from build123d import *

# Parameters (mm, degrees)
CUT_EXTRUDE_START        = -5
SKETCH_2_R               = 1.75
CUT_EXTRUDE_1_DEPTH      = 39.496268449
SKETCH_4_W               = 1.25
SKETCH_4_H               = 8
PATTERN_CIRCULAR_1_COUNT = 2
PATTERN_CIRCULAR_1_ANGLE = 90


with BuildPart() as part:
    # ｽｹｯﾁ1 → 回転1 (revolve)
    with BuildSketch(Plane.XY, mode=Mode.PRIVATE) as revolve_1_sk:
        with BuildLine():
            Line((5, 16), (5, 3))
            Line((5, 3), (-5, 3))
            Line((-5, 3), (-5, 16))
            Line((-5, 16), (-2.886751346, 16))
            Line((-2.886751346, 16), (-1.732050808, 14))
            ThreePointArc((-1.732050808, 14), (0, 13), (1.732050808, 14))
            Line((1.732050808, 14), (2.886751346, 16))
            Line((2.886751346, 16), (5, 16))
        make_face()
    revolve(revolve_1_sk.sketch.rotate(Axis((-76.157807816, 0, 0), (1, 0, 0)), 90), axis=Axis((-76.157807816, 0, 0), (1, 0, 0)))

    # ｽｹｯﾁ2 → ｶｯﾄ - 押し出し1 (cut)
    with BuildSketch(Plane(origin=(0, 13, 0), x_dir=(1, 0, 0), z_dir=(0, 1, 0)).offset(CUT_EXTRUDE_START)):
        with Locations(Location((0, 0, 0), (0, 0, 171.786783431))):
            Circle(SKETCH_2_R)
    cut_extrude_1 = extrude(amount=CUT_EXTRUDE_1_DEPTH, mode=Mode.SUBTRACT)

    # ｽｹｯﾁ4 → M3x0.5 ねじ穴1 (revolve, cut)
    with BuildSketch(Plane(origin=(0, 8, 0), x_dir=(0, 0, 1), z_dir=(1, 0, 0))):
        with Locations((0.625, 4)):
            Rectangle(SKETCH_4_W, SKETCH_4_H)
    m3x0_5_1 = revolve(axis=Axis((0, 14.35, 0), (0, -1, 0)), mode=Mode.SUBTRACT)

    # 円形ﾊﾟﾀｰﾝ1: ｶｯﾄ - 押し出し1, M3x0.5 ねじ穴1 ×2 about axis
    pattern_circular_1_axis = Axis((-88.99, 0, 0), (1, 0, 0))
    add([cut_extrude_1.rotate(pattern_circular_1_axis, i * PATTERN_CIRCULAR_1_ANGLE / (PATTERN_CIRCULAR_1_COUNT - 1)) for i in range(1, PATTERN_CIRCULAR_1_COUNT)], mode=Mode.SUBTRACT)
    add([m3x0_5_1.rotate(pattern_circular_1_axis, i * PATTERN_CIRCULAR_1_ANGLE / (PATTERN_CIRCULAR_1_COUNT - 1)) for i in range(1, PATTERN_CIRCULAR_1_COUNT)], mode=Mode.SUBTRACT)


solid = part.part
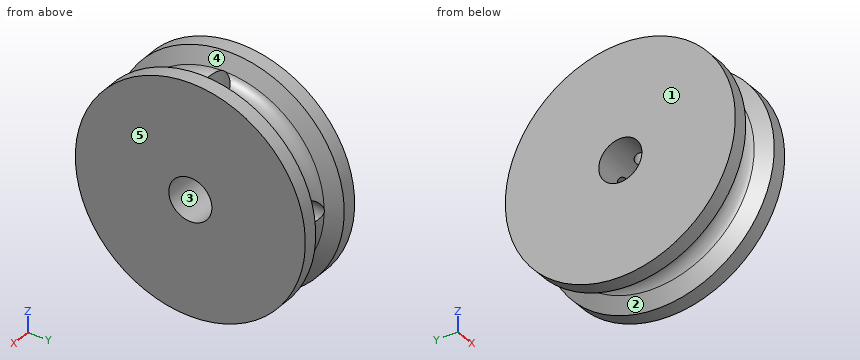
Design review of the part built by this model. Coordinates are the model's own, in mm. Face numbers are marked on the shaded views. A direction names the side the tool comes from. Coordinates: 2 decimals unless noted, no trailing zeros. Loops run counter-clockwise (first coordinate to the right, second up) from the corner with the lowest first, then second, coordinate; pieces in that order, holes last. Notation, with made-up numbers: M 11,-2.75 L 37,-2.75 A8 cw 37,2.25 Z; hole C 74,5.5 d7. An arc over 180 degrees is marked long. Answer as CSV lines item,"result".
Item 1: Machinability: for the marked faces 1 and 2, which of the approach directions +Z, -Z, +X, -X, +Y, -Y give a long, thin tool a straight path to every point of the face, cutting with its end or side? Answer none if there is none.
Answer list:
face 1,"+Z, -Z, -X, +Y, -Y"
face 2,"none"
Item 2: Add section B-B on x = 4. State the section outline as (y, z) points.
Answer list:
outline,"C 0,0 d32; hole C 0,0 d6"
Item 3: For P1, Ø3, axis at x = 0.5, z = -0.5, coming from the +Y side; P2, Ø3, axis at x = 0, y = -0.5, coming from the +Z side; P3, Ø4, axis at x = -1, y = 1.5, coming from the +Z side; P4, Ø3.5, axis at y = 0, z = 0, coming from the +X side, all flat-tipped, find the tip position at first contact; note any pin that passes through.
Answer list:
P1,"y = 14.46"
P2,"z = 13.52"
P3,"z = 15.98"
P4,"through"
Item 4: Add section A-A on x = 0. State the section outline as (y, z) points.
Answer list:
outline,"M -1.75,8 L -1.75,12.88 A13 ccw long 12.88,-1.75 L 8,-1.75 L 8,-1.25 L 2.73,-1.25 A3 cw long -1.25,2.73 L -1.25,8 Z; M 1.25,2.73 A3 cw 2.73,1.25 L 8,1.25 L 8,1.75 L 12.88,1.75 A13 ccw 1.75,12.88 L 1.75,8 L 1.25,8 Z"
Item 5: The part is to be moulded in two halves that separate along Y. For the marked faces 3, 4 and 5, say which applies: pulls with the +Y half, pulls with the -Y half, needs draft (parallel to the pull), parting line crosses it, or undercut.
Answer list:
face 3,"undercut"
face 4,"parting line crosses it"
face 5,"needs draft"
Item 6: For probe 1 along X at (y, z) = (12, 0); probe 2 along Z at (x, y) = (-1, 11.5), list the stretches that pass through material, from the lowest coordinate up.
Answer list:
probe 1,"-5 to -1.75, 1.75 to 5"
probe 2,"-6.62 to -1.44, 1.44 to 6.62"
